```python
from build123d import *

# Parameters (mm, degrees)
SKETCH1_W                           = 26.9
SKETCH1_H                           = 17.9
BOSS_EXTRUDE1_DEPTH                 = 2.54
BOSS_EXTRUDE2_DEPTH                 = 3.175
F_1_4_20_TAPPED_HOLE1_D             = 5.1054
F_1_4_20_TAPPED_HOLE1_DEPTH         = 5.715
F_3_64_0_04688_DIAMETER_HOLE1_D     = 1.190752
F_3_64_0_04688_DIAMETER_HOLE1_DEPTH = 2.54


with BuildPart() as part:
    # Sketch1 → Boss-Extrude1 (new body)
    with BuildSketch(Plane(origin=(0, 0, 0), x_dir=(1, 0, 0), z_dir=(0, 1, 0))):
        Rectangle(SKETCH1_W, SKETCH1_H)
    extrude(amount=BOSS_EXTRUDE1_DEPTH)

    # Sketch2 → Boss-Extrude2 (add)
    with BuildSketch(Plane(origin=(0, 2.54, 0), x_dir=(1, 0, 0), z_dir=(0, 1, 0))):
        with BuildLine():
            Line((-8.37, -8.95), (8.37, -8.95))
            ThreePointArc((8.37, -8.95), (10.073421181, -5.878217622), (13.45, -4.910640141))
            Line((13.45, -4.910640141), (13.45, 3.87))
            ThreePointArc((13.45, 3.87), (9.857897552, 5.357897552), (8.37, 8.95))
            Line((8.37, 8.95), (-8.37, 8.95))
            ThreePointArc((-8.37, 8.95), (-9.857897552, 5.357897552), (-13.45, 3.87))
            Line((-13.45, 3.87), (-13.45, -4.910640141))
            ThreePointArc((-13.45, -4.910640141), (-10.073421181, -5.878217622), (-8.37, -8.95))
        make_face()
    extrude(amount=BOSS_EXTRUDE2_DEPTH)

    # 1/4-20 Tapped Hole1
    with Locations(Plane(origin=(0, 5.715, 0), x_dir=(1, 0, 0), z_dir=(0, 1, 0))):
        with Locations((0, 0)):
            Hole(F_1_4_20_TAPPED_HOLE1_D / 2, depth=F_1_4_20_TAPPED_HOLE1_DEPTH)

    # 3/64 (0.04688) Diameter Hole1
    with Locations(Plane(origin=(0, 2.54, 0), x_dir=(1, 0, 0), z_dir=(0, 1, 0))):
        with Locations((-11.630674377, 7.033069438), (-11.630674377, -7.406874263), (11.813402436, -7.406874263), (11.813402436, 7.033069438)):
            Hole(F_3_64_0_04688_DIAMETER_HOLE1_D / 2, depth=F_3_64_0_04688_DIAMETER_HOLE1_DEPTH)


solid = part.part
```
Work out the finished part from the listing and answer in its coordinate system (mm). A direction names the side the tool comes from. Coordinates: 2 decimals unless noted, no trailing zeros. Order: outer loops, then holes, each group sorted by start corner. A loop starts at its lowest first (then second) coordinate and runs counter-clockwise, first axis right, second up. Notation, with made-up numbers: M -3,5.5 L 18,5.5 A14 cw 18,20.5 Z; hole C 80.5,58.25 d7. An arc over 180 degrees is marked long. Use CSV: the item, a comma, the result in double quotes.
1) For faces 1 (the face through (11, 2.54, -7)), 2 (the face through (-3, 0, 0)), 3 (the face through (-12, 2.54, -6)), 4 (the face through (11, 2.54, 7)), determine the directions among +Z, -Z, +X, -X, +Y, -Y from which every point of the face is accessible in a straight line to the end or side of a thin tool.
Worked out:
face 1,"-Z, +X, +Y"
face 2,"+Z, -Z, +X, -X, -Y"
face 3,"-Z, -X, +Y"
face 4,"+Z, +X, +Y"
2) Flat-ended cylindrical pins translate along their axes: pin 1 Ø1.2 at (x, z) = (-12, 6) entering from +Y; pin 2 Ø1.1 at (x, z) = (11.81, -7.03) entering from +Y. Find the tip coordinate at first contact, or state that the pin passes through.
Worked out:
pin 1,"stops at y = 2.54"
pin 2,"passes through"
3) Section B-B on z = 0 is taken. Write down the section's boundary in (x, y) (3 decimals), plus the area to 3 significant figures.
Worked out:
outline,"M -13.45,0 L -2.553,0 L -2.553,5.715 L -13.45,5.715 Z; M 2.553,0 L 13.45,0 L 13.45,5.715 L 2.553,5.715 Z"
area,"125 mm^2"
4) Determine the mould class of faces 5 (the face through (-9.819, 4.105, -5.398)), 6 (the face through (13.45, 2, 0)), 7 (the face through (-11.16, 1.25, 7.77)), 8 (the face through (0, 2, -8.95)) for opening direction X: released by +X, released by -X, zero draft, split by the parting line, or undercut.
Worked out:
face 5,"released by -X"
face 6,"released by +X"
face 7,"undercut"
face 8,"zero draft"
5) Section D-D on y = 1.35 is taken. Write down the section's boundary in (x, z), plus the area to 3 significant figures.
Worked out:
outline,"M -13.45,-8.95 L 13.45,-8.95 L 13.45,8.95 L -13.45,8.95 Z; hole C -11.63,-7.03 d1.19; hole C -11.63,7.41 d1.19; hole C 0,0 d5.11; hole C 11.81,-7.03 d1.19; hole C 11.81,7.41 d1.19"
area,"457 mm^2"
6) Consider line 1 (Z direction, x = 0, y = 1.2); line 2 (X direction, y = 2.45, z = -1.25); line 3 (X direction, y = 3.2, z = -1.5). Determine where each line is inside the solid, lowest interval first. Write a range as [from, to].
Worked out:
line 1,"z = [-8.95, -2.55], [2.55, 8.95]"
line 2,"x = [-13.45, -2.23], [2.23, 13.45]"
line 3,"x = [-13.45, -2.07], [2.07, 13.45]"
7) Section A-A on x = 0 is taken. Write down the section's boundary in (y, z) (3 decimals), plus the area to 3 significant figures.
Worked out:
outline,"M 0,-8.95 L 5.715,-8.95 L 5.715,-2.553 L 0,-2.553 Z; M 0,2.553 L 5.715,2.553 L 5.715,8.95 L 0,8.95 Z"
area,"73.1 mm^2"
8) Section C-C on y = 3.3 is taken. Write down the section's boundary in (x, z), plus the area to 3 significant figures.
Worked out:
outline,"M -13.45,-3.87 A5.08 cw -8.37,-8.95 L 8.37,-8.95 A5.08 cw 13.45,-3.87 L 13.45,4.91 A4.59 cw 8.37,8.95 L -8.37,8.95 A4.59 cw -13.45,4.91 Z; hole C 0,0 d5.11"
area,"388 mm^2"
